Model file for the job. Use its own axes, mm. Face numbers are marked on the shaded views. A direction names the side the tool comes from. Round coordinates to 2 decimals unless told otherwise and drop trailing zeros. Loops run counter-clockwise (first coordinate to the right, second up) from the corner with the lowest first, then second, coordinate; pieces in that order, holes last. Notation, with made-up numbers: M 3.5,50 L 42.5,50 A18 cw 42.5,79 Z; hole C 78.5,22.25 d1. An arc over 180 degrees is marked long. Answer in a Markdown table with one row per item.
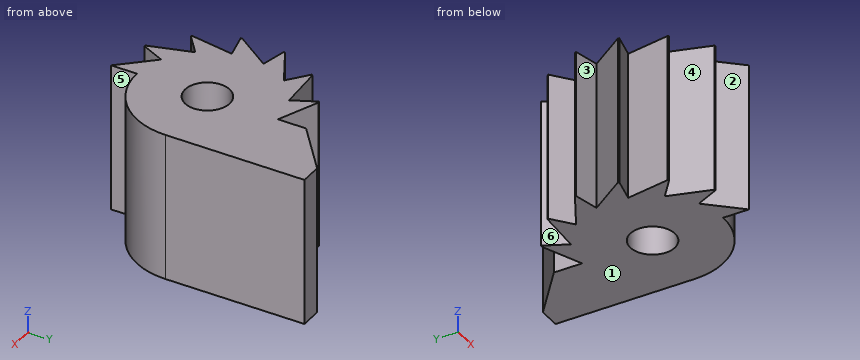
from build123d import *

# Parameters (mm, degrees)
SKETCH1_R           = 3.302
BOSS_EXTRUDE1_DEPTH = 21.971
CUT_EXTRUDE1_DEPTH  = 22.971
CUT_EXTRUDE2_DEPTH  = 22.971


with BuildPart() as part:
    # Sketch1 → Boss-Extrude1 (new body)
    with BuildSketch(Plane.XY):
        with BuildLine():
            ThreePointArc((0, -10.4775), (7.4087113, -7.4087113), (10.4775, 0))
            Line((10.4775, 0), (10.4775, 20.629972189))
            Line((10.4775, 20.629972189), (7.3025, 20.629972189))
            Line((7.3025, 20.629972189), (-0.463735424, 14.279972189))
            ThreePointArc((-0.463735424, 14.279972189), (-14.285617923, -0.23189826), (0, -14.2875))
            Line((0, -14.2875), (0, -10.4775))
        make_face()
        Circle(SKETCH1_R, mode=Mode.SUBTRACT)
    extrude(amount=BOSS_EXTRUDE1_DEPTH)

    # Sketch3 → Cut-Extrude1 (cut, through all)
    with BuildSketch(Plane.XY.offset(21.971)):
        with BuildLine():
            Line((0, -14.2875), (-4.427982837, -9.495839839))
            Line((-4.427982837, -9.495839839), (-6.038158415, -12.948872507))
            ThreePointArc((-6.038158415, -12.948872507), (-3.092380984, -13.948829202), (0, -14.2875))
        make_face()
        with BuildLine():
            Line((-8.12333208, -6.617362176), (-11.077271018, -9.023675694))
            ThreePointArc((-11.077271018, -9.023675694), (-8.861614581, -11.207338813), (-6.225846847, -12.859684572))
            Line((-6.225846847, -12.859684572), (-8.12333208, -6.617362176))
        make_face()
        with BuildLine():
            Line((-10.195077632, -2.416277786), (-13.902378588, -3.294924253))
            ThreePointArc((-13.902378588, -3.294924253), (-12.859684572, -6.225846847), (-11.207338813, -8.861614581))
            Line((-11.207338813, -8.861614581), (-10.195077632, -2.416277786))
        make_face()
        with BuildLine():
            Line((-10.229141415, 2.267746055), (-13.948829202, 3.092380984))
            ThreePointArc((-13.948829202, 3.092380984), (-14.2875, 0), (-13.948829202, -3.092380984))
            Line((-13.948829202, -3.092380984), (-10.229141415, 2.267746055))
        make_face()
        with BuildLine():
            Line((-8.218715129, 6.49851736), (-11.207338813, 8.861614581))
            ThreePointArc((-11.207338813, 8.861614581), (-12.859684572, 6.225846847), (-13.902378588, 3.294924253))
            Line((-13.902378588, 3.294924253), (-8.218715129, 6.49851736))
        make_face()
        with BuildLine():
            Line((-4.565621021, 9.430435353), (-6.225846847, 12.859684572))
            ThreePointArc((-6.225846847, 12.859684572), (-8.861614581, 11.207338813), (-11.077271018, 9.023675694))
            Line((-11.077271018, 9.023675694), (-4.565621021, 9.430435353))
        make_face()
        with BuildLine():
            Line((0, 10.4775), (0, 14.2875))
            ThreePointArc((0, 14.2875), (-3.092380984, 13.948829202), (-6.038158415, 12.948872507))
            Line((-6.038158415, 12.948872507), (0, 10.4775))
        make_face()
    extrude(amount=-CUT_EXTRUDE1_DEPTH, mode=Mode.SUBTRACT)

    # Sketch4 → Cut-Extrude2 (cut, through all)
    with BuildSketch(Plane.XY.offset(21.971)):
        Polygon((-0.463735424, 14.279972189), (0, 14.2875), (0, 14.659141732), align=None)
    extrude(amount=-CUT_EXTRUDE2_DEPTH, mode=Mode.SUBTRACT)


solid = part.part
1. Saw through at B-B (x = -1.5). Write the cut outline in (y, z).
Verdict:
| item | result |
|---|---|
| outline | M -12.66,0 L -2.94,0 L -2.94,21.97 L -12.66,21.97 Z; M 2.94,0 L 11.09,0 L 11.09,21.97 L 2.94,21.97 Z |
2. Tool access for the marked faces 4, 5 and 6: list every direction of +Z, -Z, +X, -X, +Y, -Y with a clear straight run to the whole face (end or side of a thin tool).
Verdict:
| item | result |
|---|---|
| face 4 | +Z, -Z, -Y |
| face 5 | +Z, -Z, +X, -Y |
| face 6 | +Z, -Z, -X |
3. Mould opens along X. For the marked faces 1, 2 and 3 say: +X half, -X half, draft (parallel to the pull), parting line (faces both ways), or undercut.
Verdict:
| item | result |
|---|---|
| face 1 | draft |
| face 2 | undercut |
| face 3 | -X half |
4. Saw through at D-D (x = 5). Write the cut outline in (y, z).
Verdict:
| item | result |
|---|---|
| outline | M -9.21,0 L 18.75,0 L 18.75,21.97 L -9.21,21.97 Z |
5. Saw through at C-C (y = -1.5). Write the cut outline in (x, z).
Verdict:
| item | result |
|---|---|
| outline | M -12.84,0 L -2.94,0 L -2.94,21.97 L -12.84,21.97 Z; M 2.94,0 L 10.37,0 L 10.37,21.97 L 2.94,21.97 Z |
6. Pin check, flat tips, straight feed: pin 1 (1 mm diameter, centred on x = -5, y = 15, fed in from +Z); pin 2 (1 mm diameter, centred on x = -6, z = 6.5, fed in from -Y); pin 3 (3 mm diameter, centred on y = -12.5, z = 7, fed in from +X); pin 4 (10 mm diameter, centred on y = -7.5, z = 15, fed in from -X). Stop position of each tip, or through.
Verdict:
| item | result |
|---|---|
| pin 1 | passes through |
| pin 2 | stops at y = -12.95 |
| pin 3 | stops at x = 0 |
| pin 4 | stops at x = -13.95 |
7. Wall check: probe 1 along X at (y, z) = (-11.5, 4); probe 2 along Y at (x, z) = (-5, 15.75); probe 3 along Y at (x, z) = (-1.5, 8). Give the ranges that are in metal, low to high.
Verdict:
| item | result |
|---|---|
| probe 1 | x = -6.64 to -5.36, -2.58 to 0 |
| probe 2 | y = -10.72 to 9.4, 10.33 to 12.52 |
| probe 3 | y = -12.66 to -2.94, 2.94 to 11.09 |
